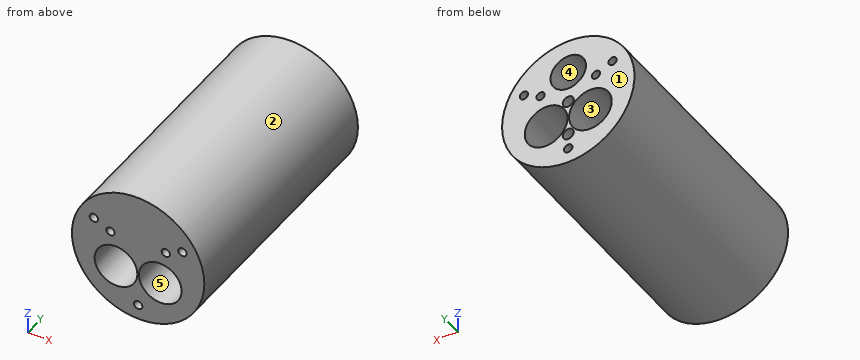
from build123d import *

# Parameters (mm, degrees)
SKETCH1_R               = 37.973
BOSS_EXTRUDE1_DEPTH     = 142.8496
SKETCH2_R               = 2.413
CUT_EXTRUDE1_DEPTH      = 143.8496
SKETCH3_R               = 12.2555
CUT_EXTRUDE2_DEPTH      = 143.8496
SKETCH4_R               = 3.175
CUT_EXTRUDE3_DEPTH      = 6.35
SKETCH5_R               = 10.16
CUT_EXTRUDE4_DEPTH      = 17.78
SKETCH6_R               = 2.38125
CUT_EXTRUDE5_DEPTH      = 1
CUT_EXTRUDE5_DEPTH_BACK = 143.8496


with BuildPart() as part:
    # Sketch1 → Boss-Extrude1 (new body)
    with BuildSketch(Plane(origin=(0, 0, 0), x_dir=(1, 0, 0), z_dir=(0, 1, 0))):
        Circle(SKETCH1_R)
    extrude(amount=BOSS_EXTRUDE1_DEPTH)

    # Sketch2 → Cut-Extrude1 (cut, through all)
    with BuildSketch(Plane(origin=(0, 142.8496, 0), x_dir=(1, 0, 0), z_dir=(0, 1, 0))):
        with Locations((0, 29.337)):
            Circle(SKETCH2_R)
        with Locations((25.406587271, -14.6685)):
            Circle(SKETCH2_R)
        with Locations((-25.406587271, -14.6685)):
            Circle(SKETCH2_R)
    extrude(amount=-CUT_EXTRUDE1_DEPTH, mode=Mode.SUBTRACT)

    # Sketch3 → Cut-Extrude2 (cut, through all)
    with BuildSketch(Plane(origin=(0, 142.8496, 0), x_dir=(1, 0, 0), z_dir=(0, 1, 0))):
        with Locations((-12.7, 10.16)):
            Circle(SKETCH3_R)
        with Locations((12.7, 10.16)):
            Circle(SKETCH3_R)
    extrude(amount=-CUT_EXTRUDE2_DEPTH, mode=Mode.SUBTRACT)

    # Sketch4 → Cut-Extrude3 (cut)
    with BuildSketch(Plane(origin=(0, 142.8496, 0), x_dir=(1, 0, 0), z_dir=(0, 1, 0))):
        with Locations((0, 20.32)):
            Circle(SKETCH4_R)
        Circle(SKETCH4_R)
    extrude(amount=-CUT_EXTRUDE3_DEPTH, mode=Mode.SUBTRACT)

    # Sketch5 → Cut-Extrude4 (cut)
    with BuildSketch(Plane(origin=(0, 142.8496, 0), x_dir=(1, 0, 0), z_dir=(0, 1, 0))):
        with Locations((0, -18.415)):
            Circle(SKETCH5_R)
    extrude(amount=-CUT_EXTRUDE4_DEPTH, mode=Mode.SUBTRACT)

    # Sketch6 → Cut-Extrude5 (cut, two sides)
    with BuildSketch(Plane(origin=(0, 142.8496, 0), x_dir=(1, 0, 0), z_dir=(0, 1, 0))) as cut_extrude5_sk:
        with Locations((15.875, -10.16)):
            Circle(SKETCH6_R)
        with Locations((-15.875, -10.16)):
            Circle(SKETCH6_R)
    extrude(amount=CUT_EXTRUDE5_DEPTH, mode=Mode.SUBTRACT)
    extrude(cut_extrude5_sk.sketch, amount=-CUT_EXTRUDE5_DEPTH_BACK, mode=Mode.SUBTRACT)


solid = part.part
The listing builds one solid part. Answer for the finished solid, in the listing's coordinates (mm). Face numbers are marked on the shaded views. A direction names the side the tool comes from. Coordinates: 2 decimals unless noted, no trailing zeros. Order: outer loops, then holes, each group sorted by start corner. A loop starts at its lowest first (then second) coordinate and runs counter-clockwise, first axis right, second up. Notation, with made-up numbers: (-33, 44.5) -> (12, 44.5) arc R18 ccw to (12, 79.5) -> close; hole circle Ø5 at (2.25, 77.25). An arc over 180 degrees is marked (long way). Answer in a Markdown table with one row per item. Add a question column.
Item 1: Each of these flat-tipped pins is pushed along its axis until it touches: P1, Ø3, axis at x = -1, z = 0.5, coming from the +Y side; P2, Ø2, axis at y = 28, z = -15.5, coming from the -X side; P3, Ø7.5, axis at x = 25.41, z = 14.67, coming from the +Y side; P4, Ø4, axis at x = 8, y = 84.5, coming from the +Z side. Where does it stop, or does it pass through?
Item 2: Determine the mould class of the marked faces 1, 2 and 3 for opening direction Z: +Z half, -Z half, draft (parallel to the pull), parting line (faces both ways), or undercut.
Item 3: Find section B-B (z = -10.16). Write down the section's boundary in (x, y), then the cut area to 3 significant figures.
Item 4: Find section C-C (y = 68). Write down the section's boundary in (x, z) (1 decimal).
Item 5: Find section D-D (z = 10.16). Write down the section's boundary in (x, y), then the cut area to 3 significant figures.
Item 6: Find section A-A (x = 7.5). Write down the section's boundary in (y, z).
Item 7: Find the intervals of material crossed by L1, parallel to Z at x = 0, y = 139 (3 decimals); L2, parallel to Z at x = 0, y = 132.5 (3 decimals); L3, parallel to X at y = 141, z = -20.32 (3 decimals), in increasing order. Write a range as from..to.
Item 8: Which of the six approach directions +Z, -Z, +X, -X, +Y, -Y give full straight-line access (tool end or side, diameter ignored) to the marked faces 4 and 5?
Result set:
| question | item | result |
|---|---|---|
| 1 | P1 | stops at y = 136.5 |
| 1 | P2 | stops at x = -35.1 |
| 1 | P3 | stops at y = 142.85 |
| 1 | P4 | stops at z = 37.5 |
| 2 | face 1 | draft |
| 2 | face 2 | parting line |
| 2 | face 3 | undercut |
| 3 | outline | (-36.59, 0) -> (-24.96, 0) -> (-24.96, 142.85) -> (-36.59, 142.85) -> close; (-0.44, 0) -> (0.44, 0) -> (0.44, 142.85) -> (-0.44, 142.85) -> close; (24.96, 0) -> (36.59, 0) -> (36.59, 142.85) -> (24.96, 142.85) -> close |
| 3 | area | 3,450 mm² |
| 4 | outline | circle Ø75.9 at (0, 0); hole circle Ø4.8 at (-25.4, 14.7); hole circle Ø24.5 at (-12.7, -10.2); hole circle Ø4.8 at (-15.9, 10.2); hole circle Ø4.8 at (0, -29.3); hole circle Ø24.5 at (12.7, -10.2); hole circle Ø4.8 at (15.9, 10.2); hole circle Ø4.8 at (25.4, 14.7) |
| 5 | outline | (-36.59, 0) -> (-18.26, 0) -> (-18.26, 142.85) -> (-36.59, 142.85) -> close; (-13.49, 0) -> (13.49, 0) -> (13.49, 142.85) -> (5.92, 142.85) -> (5.92, 125.07) -> (-5.92, 125.07) -> (-5.92, 142.85) -> (-13.49, 142.85) -> close; (18.26, 0) -> (36.59, 0) -> (36.59, 142.85) -> (18.26, 142.85) -> close |
| 5 | area | 8,880 mm² |
| 6 | outline | (0, -37.22) -> (142.85, -37.22) -> (142.85, -21.26) -> (0, -21.26) -> close; (0, 0.94) -> (142.85, 0.94) -> (142.85, 11.56) -> (125.07, 11.56) -> (125.07, 25.27) -> (142.85, 25.27) -> (142.85, 37.22) -> (0, 37.22) -> close |
| 7 | L1 | z = -37.973..-31.75, -26.924..-23.495, -17.145..-3.175, 3.175..8.255, 28.575..37.973 |
| 7 | L2 | z = -37.973..-31.75, -26.924..8.255, 28.575..37.973 |
| 7 | L3 | x = -32.079..-19.554, -5.846..-3.175, 3.175..5.846, 19.554..32.079 |
| 8 | face 4 | +Y |
| 8 | face 5 | +Y, -Y |
